```python
from build123d import *

# Parameters (mm, degrees)
IZIM1_W                     = 60
IZIM1_H                     = 30
Y_KSEKLIK_EKSTR_ZYON1_DEPTH = 30
KES_EKSTR_ZYON1_DEPTH       = 30
IZIM3_W                     = 60.882003546
IZIM3_H                     = 31.045979635
KES_EKSTR_ZYON2_DEPTH       = 68
IZIM5_R                     = 1.5
KES_EKSTR_ZYON3_DEPTH       = 68
IZIM6_W                     = 6
IZIM6_H                     = 30
KES_EKSTR_ZYON6_DEPTH       = 68
KES_EKSTR_ZYON6_DEPTH_BACK  = 68
IZIM7_R                     = 1.5
KES_EKSTR_ZYON7_DEPTH       = 68
IZIM8_W                     = 21.364552878
IZIM8_H                     = 18
KES_EKSTR_ZYON8_DEPTH       = 68
KES_EKSTR_ZYON9_DEPTH       = 68
KES_EKSTR_ZYON10_DEPTH      = 68
KES_EKSTR_ZYON11_DEPTH      = 68
KES_EKSTR_ZYON12_DEPTH      = 68


with BuildPart() as part:
    # izim1 → Y_kseklik-Ekstr_zyon1 (new body)
    with BuildSketch(Plane(origin=(0, 0, 0), x_dir=(1, 0, 0), z_dir=(0, 1, 0))):
        with Locations((2.921722845, -2.96539542)):
            Rectangle(IZIM1_W, IZIM1_H)
    extrude(amount=Y_KSEKLIK_EKSTR_ZYON1_DEPTH)

    # izim2 → Kes-Ekstr_zyon1 (cut)
    with BuildSketch(Plane.XY.offset(17.96539542)):
        Polygon((-27.078277155, 0), (32.921722845, 30), (-27.078277155, 30), align=None)
    extrude(amount=-KES_EKSTR_ZYON1_DEPTH, mode=Mode.SUBTRACT)

    # izim3 → Kes-Ekstr_zyon2 (cut)
    with BuildSketch(Plane.XY.offset(17.96539542)):
        with Locations((-1.054812834, 19.120649243)):
            Rectangle(IZIM3_W, IZIM3_H)
    extrude(amount=-KES_EKSTR_ZYON2_DEPTH, mode=Mode.SUBTRACT)

    # izim5 → Kes-Ekstr_zyon3 (cut)
    with BuildSketch(Plane.ZY.offset(-29.386188939)):
        with Locations((2.96539542, 15.914946236)):
            Circle(IZIM5_R)
    extrude(amount=-KES_EKSTR_ZYON3_DEPTH, mode=Mode.SUBTRACT)

    # izim6 → Kes-Ekstr_zyon6 (cut, two sides)
    with BuildSketch(Plane.ZY.offset(-29.386188939)) as kes_ekstr_zyon6_sk:
        with Locations((-9.03460458, 15)):
            Rectangle(IZIM6_W, IZIM6_H)
        with Locations((14.96539542, 15)):
            Rectangle(IZIM6_W, IZIM6_H)
    extrude(amount=KES_EKSTR_ZYON6_DEPTH, mode=Mode.SUBTRACT)
    extrude(kes_ekstr_zyon6_sk.sketch, amount=-KES_EKSTR_ZYON6_DEPTH_BACK, mode=Mode.SUBTRACT)

    # izim7 → Kes-Ekstr_zyon7 (cut)
    with BuildSketch(Plane(origin=(0, 3.597659425, 0), x_dir=(1, 0, 0), z_dir=(0, 1, 0))):
        with Locations((6.51938227, -2.96539542)):
            Circle(IZIM7_R)
    extrude(amount=-KES_EKSTR_ZYON7_DEPTH, mode=Mode.SUBTRACT)

    # izim8 → Kes-Ekstr_zyon8 (cut)
    with BuildSketch(Plane(origin=(0, 3.597659425, 0), x_dir=(1, 0, 0), z_dir=(0, 1, 0))):
        with Locations((-16.396000716, -2.96539542)):
            Rectangle(IZIM8_W, IZIM8_H)
    extrude(amount=-KES_EKSTR_ZYON8_DEPTH, mode=Mode.SUBTRACT)

    # izim9 → Kes-Ekstr_zyon9 (cut)
    with BuildSketch(Plane.XY.offset(11.96539542)):
        Polygon((-5.713724277, 3.597659425), (-2.116064853, 0), (-5.713724277, 0), align=None)
    extrude(amount=-KES_EKSTR_ZYON9_DEPTH, mode=Mode.SUBTRACT)

    # izim10 → Kes-Ekstr_zyon10 (cut)
    with BuildSketch(Plane.XY.offset(11.96539542)):
        Polygon((29.386188939, 28.232233047), (32.921722845, 24.696699141), (29.386188939, 24.696699141), align=None)
    extrude(amount=-KES_EKSTR_ZYON10_DEPTH, mode=Mode.SUBTRACT)

    # izim11 → Kes-Ekstr_zyon11 (cut)
    with BuildSketch(Plane.XY.offset(11.96539542)):
        Polygon((29.386188939, 28.232233047), (32.921722845, 30), (32.921722845, 24.696699141), align=None)
    extrude(amount=-KES_EKSTR_ZYON11_DEPTH, mode=Mode.SUBTRACT)

    # izim12 → Kes-Ekstr_zyon12 (cut)
    with BuildSketch(Plane.XY.offset(11.96539542)):
        Polygon((29.386188939, 24.696699141), (32.921722845, 21.161165235), (32.921722845, 24.696699141), align=None)
    extrude(amount=-KES_EKSTR_ZYON12_DEPTH, mode=Mode.SUBTRACT)


solid = part.part
```
Verification items for the finished model (mm, model axes). A direction names the side the tool comes from. Coordinates: 2 decimals unless noted, no trailing zeros. Write each loop counter-clockwise with the first axis right and the second up, starting at its lowest first coordinate (ties: lowest second). Pieces come first, ordered by that corner, then holes. Notation, with made-up numbers: M -10.5,-2.5 L 34.5,-2.5 A20 cw 34.5,2.5 Z; hole C 45.25,-5 d5. An arc over 180 degrees is marked long. Answer as a JSON object with one key per item and string values. Group by question number.
(1) Cross-section at D-D, the plane y = 7.5. Record the cut outline in (x, z), and give its area (3 significant figures).
(2) Gauge pin test, flat ends, axial feed: pin 1 (10 mm diameter, centred on y = 2.5, z = 0, fed in from -X); pin 2 (9 mm diameter, centred on y = 16, z = 1.5, fed in from -X). Record the tip position at first contact, or that the pin passes through.
(3) Cross-section at A-A, the plane y = 16.75. Record the cut outline in (x, z).
(4) Release check for a two-part mould opening along Z. For faces 1 (the face through (31.129, 22.954, 3.091)), 2 (the face through (5.33, 1.82, 3.88)), 3 (the face through (19, 3, 11.965)) record: +Z half, -Z half, draft (parallel to the pull), parting line (faces both ways), or undercut.
(5) Material ranges on line 1 (X direction, y = 10.5, z = -0.75); line 2 (Y direction, x = 14, z = 6.5); line 3 (Y direction, x = 31.5, z = -2), recorded low to high.
(6) Tool access check on faces 4 (the face through (31.129, 14.584, 3.658)), 5 (the face through (12, 3.598, 3)). Record the directions out of +Z, -Z, +X, -X, +Y, -Y that give a thin tool (end or side, any length) a straight path to the whole face; none if there is none.
(7) Cross-section at C-C, the plane z = 6.75. Record the cut outline in (x, y).
(8) Cross-section at B-B, the plane x = 6. Record the cut outline in (y, z).
Reply:
{
 "1": {"outline": "M 29.39,-6.03 L 32.92,-6.03 L 32.92,11.97 L 29.39,11.97 Z", "area": "63.6 mm²"},
 "2": {"pin 1": "x = -5.71", "pin 2": "x = 29.39"},
 "3": {"outline": "M 29.39,-6.03 L 32.92,-6.03 L 32.92,1.72 L 29.39,1.72 Z; M 29.39,4.21 L 32.92,4.21 L 32.92,11.97 L 29.39,11.97 Z"},
 "4": {"face 1": "draft", "face 2": "undercut", "face 3": "+Z half"},
 "5": {"line 1": "29.39 to 32.92", "line 2": "0 to 3.6", "line 3": "0 to 22.58"},
 "6": {"face 4": "+X, -X", "face 5": "+Z, -Z, -X, +Y"},
 "7": {"outline": "M -5.71,3.6 L -2.12,0 L 32.92,0 L 32.92,21.16 L 29.39,24.7 L 29.39,3.6 Z"},
 "8": {"outline": "M 0,-6.03 L 3.6,-6.03 L 3.6,1.56 L 0,1.56 Z; M 0,4.37 L 3.6,4.37 L 3.6,11.97 L 0,11.97 Z"}
}
